Here's how the part is built. I have some questions about the finished solid (model axes, mm). A direction names the side the tool comes from. Coordinates: 2 decimals unless noted, no trailing zeros. Write each loop counter-clockwise with the first axis right and the second up, starting at its lowest first coordinate (ties: lowest second). Pieces come first, ordered by that corner, then holes. Notation, with made-up numbers: (-30, -25.75) -> (-24, -25.75) arc R28 ccw to (-24, -0.75) -> close; hole circle Ø3 at (65, 65.5). An arc over 180 degrees is marked (long way). Use a Markdown table: item, result. Add a question column.
Item 1: Imagine slicing it at B-B, the plane z = 0. Write out the boundary of the cut face in (x, y).
Item 2: Imagine slicing it at C-C, the plane y = -30.5. Write out the boundary of the cut face in (x, z).
Item 3: Imagine slicing it at D-D, the plane x = -43.5. Write out the boundary of the cut face in (y, z).
Item 4: If we mould it in two halves opening along Y, with no side actions, what happens to faces 3 (the cylindrical face through (-23.183, -2.504, 30.235)), 4 (the flat face through (0, -38.1, 0)), 5 (the flat face through (50.8, 3, -1))? For each: pulls with the +Y half, pulls with the -Y half, needs draft (parallel to the pull), parting line crosses it, or undercut.
Item 5: Imagine slicing it at A-A, the plane x = 0. Write out the boundary of the cut face in (y, z), and give its area (3 significant figures).
Item 6: Will these pins go through, and if not, where does the flat tip stop? pin 1 Ø1 at (y, z) = (-30, 8.5) entering from +X; pin 2 Ø1 at (x, z) = (-30, -39) entering from -Y; pin 3 Ø8 at (y, z) = (-0.5, 29) entering from +X; pin 4 Ø8 at (y, z) = (-10.5, 0.5) entering from -X.
Item 7: If I drill on line 1 along Y through (x, z) = (-17, -42); line 2 along X through (y, z) = (-25, -0.5); line 3 along Y through (x, z) = (-28, -25), over which ranges is the centre line in solid material (lowest first)? Write a range as from..to.
Item 8: On a 3-axis mill with a long thin cutter (end or side, diameter ignored), from which of +Z, -Z, +X, -X, +Y, -Y can I reach the whole of each face in a straight line? I mean faces 1 (the cylindrical face through (7.555, -23.446, 0.992)), 2 (the cylindrical face through (-46.799, 2.504, 47.006)). Say none if no direction works.
```python
from build123d import *

# Parameters (mm, degrees)
BOSS_EXTRUDE1_DEPTH = 5.08
SKETCH2_R           = 38.1
BOSS_EXTRUDE2_DEPTH = 10.16
SKETCH3_R           = 2.54
SKETCH5_R           = 7.62
BOSS_EXTRUDE3_DEPTH = 27.94
CHAMFER4_SIZE       = 0.9906


with BuildPart() as part:
    # Sketch1 → Boss-Extrude1 (new body)
    with BuildSketch(Plane(origin=(0, 0, 0), x_dir=(1, 0, 0), z_dir=(0, 1, 0))):
        with BuildLine():
            Line((-37.495119859, 50.8), (37.495119859, 50.8))
            ThreePointArc((37.495119859, 50.8), (46.90309083, 46.90309083), (50.8, 37.495119859))
            Line((50.8, 37.495119859), (50.8, -37.495119859))
            ThreePointArc((50.8, -37.495119859), (46.90309083, -46.90309083), (37.495119859, -50.8))
            Line((37.495119859, -50.8), (-37.495119859, -50.8))
            ThreePointArc((-37.495119859, -50.8), (-46.90309083, -46.90309083), (-50.8, -37.495119859))
            Line((-50.8, -37.495119859), (-50.8, 37.495119859))
            ThreePointArc((-50.8, 37.495119859), (-46.90309083, 46.90309083), (-37.495119859, 50.8))
        make_face()
    extrude(amount=BOSS_EXTRUDE1_DEPTH)

    # Sketch2 → Boss-Extrude2 (add)
    with BuildSketch(Plane.XZ):
        with Locations(Location((0, 0, 0), (0, 0, 270))):
            Circle(SKETCH2_R)
    extrude(amount=BOSS_EXTRUDE2_DEPTH)

    # Sketch3 → Revolve1 (revolve)
    with BuildSketch(Plane(origin=(0, 0, 0), x_dir=(0, 0, -1), z_dir=(1, 0, 0)), mode=Mode.PRIVATE) as revolve1_sk:
        with Locations((-38.1, -7.62)):
            Circle(SKETCH3_R)
    revolve(revolve1_sk.sketch.rotate(Axis((0, 0, 0), (0, -1, 0)), 180), axis=Axis((0, 0, 0), (0, -1, 0)))

    # Sketch5 → Boss-Extrude3 (add)
    with BuildSketch(Plane.XZ.offset(10.16)):
        with Locations(Location((0, 0, 0), (0, 0, 270))):
            Circle(SKETCH5_R)
    extrude(amount=BOSS_EXTRUDE3_DEPTH)

    # Chamfer4
    chamfer4_edges = [part.edges().sort_by_distance(p)[0] for p in [
        (0, -38.1, 7.62),
    ]]
    chamfer(chamfer4_edges, length=CHAMFER4_SIZE)


solid = part.part
```
Ans:
| question | item | result |
|---|---|---|
| 1 | outline | (-50.8, 0) -> (-38.1, 0) -> (-38.1, -5.08) arc R2.54 ccw to (-38.1, -10.16) -> (-7.62, -10.16) -> (-7.62, -37.11) -> (-6.63, -38.1) -> (6.63, -38.1) -> (7.62, -37.11) -> (7.62, -10.16) -> (38.1, -10.16) arc R2.54 ccw to (38.1, -5.08) -> (38.1, 0) -> (50.8, 0) -> (50.8, 5.08) -> (-50.8, 5.08) -> close |
| 2 | outline | circle Ø15.24 at (0, 0) |
| 3 | outline | (0, -49.37) -> (5.08, -49.37) -> (5.08, 49.37) -> (0, 49.37) -> close |
| 4 | face 3 | undercut |
| 4 | face 4 | pulls with the -Y half |
| 4 | face 5 | needs draft |
| 5 | outline | (-38.1, -6.63) -> (-37.11, -7.62) -> (-10.16, -7.62) -> (-10.16, -38.1) arc R2.54 ccw to (-5.08, -38.1) -> (0, -38.1) -> (0, -50.8) -> (5.08, -50.8) -> (5.08, 50.8) -> (0, 50.8) -> (0, 38.1) -> (-5.08, 38.1) arc R2.54 ccw to (-10.16, 38.1) -> (-10.16, 7.62) -> (-37.11, 7.62) -> (-38.1, 6.63) -> close |
| 5 | area | 1,740 mm^2 |
| 6 | pin 1 | passes through |
| 6 | pin 2 | stops at y = 0 |
| 6 | pin 3 | stops at x = 50.8 |
| 6 | pin 4 | stops at x = -40.64 |
| 7 | line 1 | y = 0..5.08 |
| 7 | line 2 | x = -7.6..7.6 |
| 7 | line 3 | y = -10.16..5.08 |
| 8 | face 1 | -Y |
| 8 | face 2 | +Z, -X, +Y, -Y |
